```python
from build123d import *

# Parameters (mm, degrees)
BOSS_EXTRUDE1_DEPTH = 0.6
SKETCH14_R          = 1.6
SKETCH14_W          = 0.8
SKETCH14_H          = 30.7
SKETCH14_H_2        = 16.55
SKETCH14_H_3        = 17.4
SKETCH14_H_4        = 18.55
SKETCH14_H_5        = 16
CUT_EXTRUDE1_DEPTH  = 1.6
FILLET3_R           = 6
SKETCH15_R          = 1.6
CUT_EXTRUDE2_DEPTH  = 1.6
SKETCH16_W          = 25
SKETCH16_H          = 5
BOSS_EXTRUDE2_DEPTH = 0.6
SKETCH17_W          = 9.2
SKETCH17_H          = 0.8
CUT_EXTRUDE3_DEPTH  = 1.6
FILLET4_R           = 3


with BuildPart() as part:
    # Sketch2 → Boss-Extrude1 (new body)
    with BuildSketch(Plane.XY):
        Polygon((106.16728925, 147.241288665), (106.16728925, 31.58105), (24.16705825, 31.58105), (-10.832812, 31.58105), (-10.832812, 185.1806075), (24.16705825, 185.1806075), (106.16728925, 185.1806075), (111.16728925, 185.1806075), (111.16728925, 147.241288665), align=None)
    extrude(amount=BOSS_EXTRUDE1_DEPTH)

    # Sketch14 → Cut-Extrude1 (cut, through all)
    with BuildSketch(Plane.XY.offset(0.6)):
        with Locations((100.166839875, 36.181495)):
            Circle(SKETCH14_R)
        with Locations((8.167632375, 36.181495)):
            Circle(SKETCH14_R)
        with Locations((8.167632375, 151.18016)):
            Circle(SKETCH14_R)
        with Locations((100.166839875, 151.18016)):
            Circle(SKETCH14_R)
        with Locations((-5.432812, 158.23105)):
            Rectangle(SKETCH14_W, SKETCH14_H)
        with Locations((-5.432812, 50.85605)):
            Rectangle(SKETCH14_W, SKETCH14_H_2)
        with Locations((-5.432812, 131.58105)):
            Rectangle(SKETCH14_W, SKETCH14_H_3)
        with Locations((-5.432812, 71.00605)):
            Rectangle(SKETCH14_W, SKETCH14_H_4)
        with Locations((-5.432812, 91.58105)):
            Rectangle(SKETCH14_W, SKETCH14_H_3)
        with Locations((-5.432812, 111.58105)):
            Rectangle(SKETCH14_W, SKETCH14_H_3)
        with Locations((105.76728925, 165.58105)):
            Rectangle(SKETCH14_W, SKETCH14_H_5)
    extrude(amount=-CUT_EXTRUDE1_DEPTH, mode=Mode.SUBTRACT)

    # Fillet3
    fillet3_edges = [part.edges().sort_by_distance(p)[0] for p in [
        (111.16728925, 185.1806075, 0.3),
        (-10.832812, 31.58105, 0.3),
        (-10.832812, 185.1806075, 0.3),
    ]]
    fillet(fillet3_edges, radius=FILLET3_R)

    # Sketch15 → Cut-Extrude2 (cut, through all)
    with BuildSketch(Plane.XY.offset(0.6)):
        with Locations((74.166839875, 52.181495)):
            Circle(SKETCH15_R)
        with Locations((40.166839875, 42.181495)):
            Circle(SKETCH15_R)
    extrude(amount=-CUT_EXTRUDE2_DEPTH, mode=Mode.SUBTRACT)

    # Sketch16 → Boss-Extrude2 (add)
    with BuildSketch(Plane.XY.offset(0.6)):
        with Locations((50.16728925, 187.6806075)):
            Rectangle(SKETCH16_W, SKETCH16_H)
    extrude(amount=-BOSS_EXTRUDE2_DEPTH)

    # Sketch17 → Cut-Extrude3 (cut, through all)
    with BuildSketch(Plane.XY.offset(0.6)):
        with Locations((50.16728925, 184.7806075)):
            Rectangle(SKETCH17_W, SKETCH17_H)
    extrude(amount=-CUT_EXTRUDE3_DEPTH, mode=Mode.SUBTRACT)

    # Fillet4
    fillet4_edges = [part.edges().sort_by_distance(p)[0] for p in [
        (111.16728925, 147.241288665, 0.3),
        (37.66728925, 190.1806075, 0.3),
        (62.66728925, 190.1806075, 0.3),
    ]]
    fillet(fillet4_edges, radius=FILLET4_R)


solid = part.part
```
Check sheet for the modelled part. Datum: model origin and axes. Units: mm. Round coordinates to 2 decimals unless told otherwise and drop trailing zeros. Order: outer loops, then holes, each group sorted by start corner. A loop starts at its lowest first (then second) coordinate and runs counter-clockwise, first axis right, second up. Notation, with made-up numbers: (45.5, 82) -> (78.5, 82) arc R18 ccw to (78.5, 104) -> close; hole circle Ø2 at (84, 74.25). An arc over 180 degrees is marked (long way). Use CSV: the item, a comma, the result in double quotes.
(1) Cross-section at B-B (x = 94.5). Record the boundary of the cut face in (y, z).
Worked out:
outline,"(31.58, 0) -> (185.18, 0) -> (185.18, 0.6) -> (31.58, 0.6) -> close"
(2) Cross-section at C-C (z = 0.3). Count the separate pieces of the cut face and the enclosed holes in it, and give its area (3 significant figures).
Worked out:
separate pieces,"1"
enclosed holes,"14"
area,"18,100 mm²"
(3) Material ranges on line 1 along X through (y, z) = (160, 0.2); line 2 along X through (y, z) = (109, 0.1); line 3 along Y through (x, z) = (53, 0.1), recorded low to high. Write a range as from..to.
Worked out:
line 1,"-10.83..-5.83, -5.03..105.37, 106.17..111.17"
line 2,"-10.83..-5.83, -5.03..106.17"
line 3,"31.58..184.38, 185.18..190.18"
(4) Draft check along X on faces 1 (the face through (109.456, 183.376, 0.304)), 2 (the face through (51, 112, 0.6)), 3 (the face through (99.82, 149.62, 0.3)), 4 (the face through (7.82, 149.62, 0.3)). Enter one of: pulls with the +X half, pulls with the -X half, needs draft (parallel to the pull), parting line crosses it, or undercut.
Worked out:
face 1,"pulls with the +X half"
face 2,"needs draft"
face 3,"undercut"
face 4,"undercut"
(5) Cross-section at A-A (y = 85.5). Record the boundary of the cut face in (x, z), and give its area (3 significant figures).
Worked out:
outline,"(-10.83, 0) -> (-5.83, 0) -> (-5.83, 0.6) -> (-10.83, 0.6) -> close; (-5.03, 0) -> (106.17, 0) -> (106.17, 0.6) -> (-5.03, 0.6) -> close"
area,"69.7 mm²"
